Could you check a few things on this model? Use its own coordinates, in mm. A direction names the side the tool comes from. Round coordinates to 2 decimals unless told otherwise and drop trailing zeros. Write each loop counter-clockwise with the first axis right and the second up, starting at its lowest first coordinate (ties: lowest second). Pieces come first, ordered by that corner, then holes. Notation, with made-up numbers: M 46.5,5 L 61.5,5 A31 ccw 61.5,41 Z; hole C 5,60.5 d4. An arc over 180 degrees is marked long. One line per question, with ' | ' between items. Start each with the question number.
```python
from build123d import *

# Parameters (mm, degrees)
F0_R          = 12.5
F1_DEPTH      = 18
F3_R          = 12.5
F4_DEPTH      = 12
F5_R          = 12.5
F6_DEPTH      = 122
F6_DEPTH_BACK = 2


with BuildPart() as f1:
    # F0 (on Front) → F1 (new body)
    with BuildSketch(Plane.XZ):
        with BuildLine():
            Line((-26.0921634734, -100), (-26.0921634734, 0))
            Line((-26.0921634734, 0), (-302.2132738139, 0))
            ThreePointArc((-302.2132738139, 0), (-408.6771422638, -41.6946592259), (-458.5108448572, -144.6004509926))
            Line((-458.5108448572, -144.6004509926), (-145.9157027706, -144.6004509926))
            Line((-145.9157027706, -144.6004509926), (-145.9157027706, -100))
            Line((-145.9157027706, -100), (-26.0921634734, -100))
        make_face()
        with Locations((-387.568802112, -107.9307186779)):
            Circle(F0_R, mode=Mode.SUBTRACT)
        with Locations((-217.2388651936, -107.2706000321)):
            Circle(F0_R, mode=Mode.SUBTRACT)
        with Locations((-351.7133506022, -71.7962682002)):
            Circle(F0_R, mode=Mode.SUBTRACT)
        with Locations((-302.5943934917, -58.4306418896)):
            Circle(F0_R, mode=Mode.SUBTRACT)
        with Locations((-253.3733156713, -71.4151485223)):
            Circle(F0_R, mode=Mode.SUBTRACT)
    extrude(amount=F1_DEPTH)



with BuildPart() as f4:
    # F3 (on offset) → F4 (new body)
    with BuildSketch(Plane.XZ.offset(108)):
        with BuildLine():
            Line((-458.5108448572, -144.6004509926), (-145.9157027706, -144.6004509926))
            ThreePointArc((-145.9157027706, -144.6004509926), (-302.2132738139, 0), (-458.5108448572, -144.6004509926))
        make_face()
        with Locations((-387.568802112, -107.9307186779)):
            Circle(F3_R, mode=Mode.SUBTRACT)
        with Locations((-217.2388651936, -107.2706000321)):
            Circle(F3_R, mode=Mode.SUBTRACT)
        with Locations((-351.7133506022, -71.7962682002)):
            Circle(F3_R, mode=Mode.SUBTRACT)
        with Locations((-302.5943934917, -58.4306418896)):
            Circle(F3_R, mode=Mode.SUBTRACT)
        with Locations((-253.3733156713, -71.4151485223)):
            Circle(F3_R, mode=Mode.SUBTRACT)
    extrude(amount=F4_DEPTH)


with BuildPart() as f1_1:
    add(f1.part)

    add(f4.part)  # F6 merges F4
    # F5 (on face) → F6 (join, two sides)
    with BuildSketch(Plane.XZ.offset(120)) as f6_sk:
        with Locations((-387.568802112, -107.9307186779)):
            Circle(F5_R)
        with Locations((-351.7133506022, -71.7962682002)):
            Circle(F5_R)
        with Locations((-302.5943934917, -58.4306418896)):
            Circle(F5_R)
        with Locations((-253.3733156713, -71.4151485223)):
            Circle(F5_R)
        with Locations((-217.2388651936, -107.2706000321)):
            Circle(F5_R)
    extrude(amount=-F6_DEPTH)
    extrude(f6_sk.sketch, amount=F6_DEPTH_BACK)


solid = f1_1.part
```
1. I'm going to push flat-ended pins straight in: P1, Ø1, axis at x = -244, z = -115, coming from the +Y side; P2, Ø12, axis at x = -316.5, y = -96, coming from the -Z side; P3, Ø2, axis at x = -356, z = -116, coming from the -Y side; P4, Ø1.5, axis at x = -184.5, y = -19.5, coming from the +Z side. Where does each tip first touch, or does it pass through?
2. Suppose I cut it at A-A (x = -333). Write out the boundary of the cut face in (y, z), and give its area (3 significant figures).
3. Suppose I cut it at C-C (y = -9). Write out the boundary of the cut face in (x, z).
4. Suppose I cut it at B-B (z = -22). Write out the boundary of the cut face in (x, y).
5. If we mould it in two halves opening along Y, with no side actions, what happens to faces 6 (the face through (-26.092, -9, -51)), 7 (the face through (-388, -122, -108)), 8 (the face through (-265.86, -63.63, -70.87))? For each: released by +Y, released by -Y, zero draft, split by the parting line, or undercut.
6. Suppose I cut it at D-D (y = -50.5). Write out the boundary of the cut face in (x, z).
7. Which directions (+Z, -Z, +X, -X, +Y, -Y) give clear straight access to the entire face, cutting with the end or side of a thin tool? Please do faces 1 (the face through (-303, 2, -58)), 2 (the face through (-265.86, -120.99, -70.87)), 3 (the face through (-339.79, -63.63, -68.04)), 4 (the face through (-145.916, -9, -123)), 5 (the face through (-376.022, 0.986, -112.718)).
8. I need wall thicknesses on line 1 along Y through (x, z) = (-222.5, -47.5); line 2 along X through (y, z) = (-58.5, -76); line 3 along Y through (x, z) = (-110, -11.5). Which ranges of each line are inside material? Lowest first, please. Write a range as from..to.
Computed:
1) P1: stops at y = 0 | P2: stops at z = -68.11 | P3: stops at y = -120 | P4: passes through
2) outline: M -120,-144.6 L -108,-144.6 L -108,-3.05 L -120,-3.05 Z; M -18,-144.6 L 0,-144.6 L 0,-3.05 L -18,-3.05 Z | area: 4,250 mm²
3) outline: M -458.51,-144.6 L -145.92,-144.6 L -145.92,-100 L -26.09,-100 L -26.09,0 L -302.21,0 A156.77 ccw Z
4) outline: M -382.3,-120 L -222.13,-120 L -222.13,-108 L -382.3,-108 Z; M -382.3,-18 L -26.09,-18 L -26.09,0 L -382.3,0 Z
5) face 6: zero draft | face 7: released by -Y | face 8: undercut
6) outline: C -387.57,-107.93 d25; C -351.71,-71.8 d25; C -302.59,-58.43 d25; C -253.37,-71.42 d25; C -217.24,-107.27 d25
7) face 1: +Z, -Z, +X, -X, +Y | face 2: -Y | face 3: none | face 4: -Z, +X, +Y, -Y | face 5: +Y
8) line 1: y = -120..-108, -18..0 | line 2: x = -363.49..-339.94, -265..-241.74 | line 3: y = -18..0
